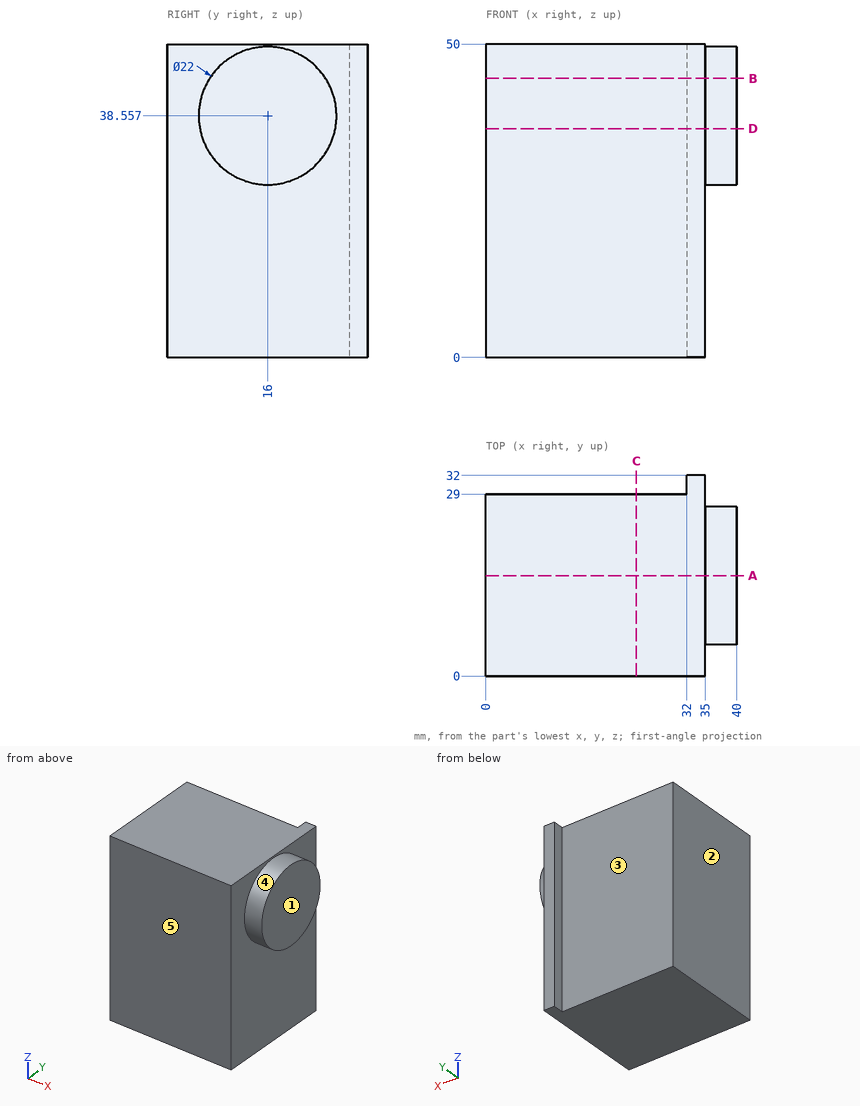
Geometry check sheet. Reference: drawing and pictorial views, mm from the part's lowest x, y, z. A direction names the side the tool comes from. Round coordinates to 2 decimals unless told otherwise and drop trailing zeros. Loops run counter-clockwise (first coordinate to the right, second up) from the corner with the lowest first, then second, coordinate; pieces in that order, holes last. Notation, with made-up numbers: (-4, -30.75) - (37, -30.75) arc R6 cw to (37, -19.75) - close; hole circle Ø10 at (63, -7). An arc over 180 degrees is marked (long way). One line per question, with ' | ' between items. Start each with the question number.
1. Cross-section at D-D on z = 36.5. Record the cut outline in (x, y).
2. Cross-section at B-B on z = 44.5. Record the cut outline in (x, y), then the cut area to 3 significant figures.
3. Draft check along X on the marked faces 1, 2 and 3. Enter one of: released by +X, released by -X, zero draft, split by the parting line, or undercut.
4. Cross-section at C-C on x = 24. Record the cut outline in (y, z).
5. Depth check by flat-ended pin: pin 1 (5 mm diameter, centred on y = 15, z = 14.5, fed in from +X); pin 2 (3 mm diameter, centred on x = 4.5, z = 45, fed in from +Y). Enter the tip coordinate at first touch or a pass-through.
6. Tool access check on the marked faces 4 and 5. Record the directions out of +Z, -Z, +X, -X, +Y, -Y that give a thin tool (end or side, any length) a straight path to the whole face; none if there is none.
7. Scan lines: line 1 (X direction, y = 18, z = 24.5); line 2 (Y direction, x = 8.5, z = 24.5); line 3 (Z direction, x = 35.5, y = 23.5). Record each from-to range of solid material in increasing order. Write a range as [from, to].
8. Cross-section at A-A on y = 16. Record the cut outline in (x, z).
Taken from the geometry:
1) outline: (0, 0) - (35, 0) - (35, 5.19) - (40, 5.19) - (40, 26.81) - (35, 26.81) - (35, 32) - (32, 32) - (32, 29) - (0, 29) - close
2) outline: (0, 0) - (35, 0) - (35, 6.74) - (40, 6.74) - (40, 25.26) - (35, 25.26) - (35, 32) - (32, 32) - (32, 29) - (0, 29) - close | area: 1,120 mm²
3) face 1: released by +X | face 2: released by -X | face 3: zero draft
4) outline: (0, 0) - (29, 0) - (29, 50) - (0, 50) - close
5) pin 1: x = 35 | pin 2: y = 29
6) face 4: +X | face 5: +Z, -Z, +X, -X, -Y
7) line 1: [0, 35] | line 2: [0, 29] | line 3: [30.51, 46.6]
8) outline: (0, 0) - (35, 0) - (35, 27.56) - (40, 27.56) - (40, 49.56) - (35, 49.56) - (35, 50) - (0, 50) - close
